from build123d import *

# Parameters (mm, degrees)
SKETCH1_W           = 13
SKETCH1_H           = 13
BOSS_EXTRUDE1_DEPTH = 85
SKETCH2_W           = 13
SKETCH2_H           = 30.5
BOSS_EXTRUDE2_DEPTH = 3
SKETCH3_R           = 2.1
CUT_EXTRUDE1_DEPTH  = 11.5
SKETCH4_R           = 5.25
CUT_EXTRUDE2_DEPTH  = 4.5


with BuildPart() as part:
    # Sketch1 → Boss-Extrude1 (new, symmetric)
    with BuildSketch(Plane.XY):
        Rectangle(SKETCH1_W, SKETCH1_H)
    extrude(amount=BOSS_EXTRUDE1_DEPTH, both=True)

    # Sketch2 → Boss-Extrude2 (add, symmetric)
    with BuildSketch(Plane.XY.offset(82)):
        with Locations((0, -20.75)):
            Rectangle(SKETCH2_W, SKETCH2_H)
    extrude(amount=BOSS_EXTRUDE2_DEPTH, both=True)

    # Sketch3 → Cut-Extrude1 (cut, symmetric)
    with BuildSketch(Plane(origin=(0, 0, 0), x_dir=(0, 0, -1), z_dir=(1, 0, 0))):
        with Locations((72.5, 0)):
            Circle(SKETCH3_R)
        with Locations((47.5, 0)):
            Circle(SKETCH3_R)
        with Locations((22.5, 0)):
            Circle(SKETCH3_R)
        with Locations((-2.5, 0)):
            Circle(SKETCH3_R)
        with Locations((-27.5, 0)):
            Circle(SKETCH3_R)
        with Locations((-52.5, 0)):
            Circle(SKETCH3_R)
        with Locations((-72.5, 0)):
            Circle(SKETCH3_R)
    extrude(amount=CUT_EXTRUDE1_DEPTH, both=True, mode=Mode.SUBTRACT)

    # Sketch4 → Cut-Extrude2 (cut, symmetric)
    with BuildSketch(Plane(origin=(-6.5, 0, 0), x_dir=(0, 0, -1), z_dir=(1, 0, 0))):
        with Locations((72.5, 0)):
            Circle(SKETCH4_R)
        with Locations((47.5, 0)):
            Circle(SKETCH4_R)
        with Locations((22.5, 0)):
            Circle(SKETCH4_R)
        with Locations((-2.5, 0)):
            Circle(SKETCH4_R)
        with Locations((-27.5, 0)):
            Circle(SKETCH4_R)
        with Locations((-52.5, 0)):
            Circle(SKETCH4_R)
        with Locations((-72.5, 0)):
            Circle(SKETCH4_R)
    extrude(amount=CUT_EXTRUDE2_DEPTH, both=True, mode=Mode.SUBTRACT)


solid = part.part
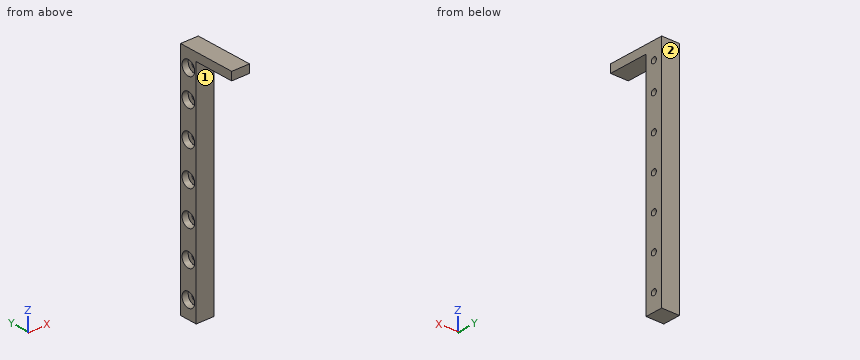
The listing builds one solid part. Answer for the finished solid, in the listing's coordinates (mm). Face numbers are marked on the shaded views. A direction names the side the tool comes from. Give positions to 0.01 mm unless a question says otherwise; leave off trailing zeros. Write each loop counter-clockwise with the first axis right and the second up, starting at its lowest first coordinate (ties: lowest second). Pieces come first, ordered by that corner, then holes. Notation, with made-up numbers: (36.25, 40) - (92.25, 40) arc R17 cw to (92.25, 65) - close; hole circle Ø8 at (-26.75, 81.25). An arc over 180 degrees is marked (long way). One line per question, with ' | ' between items. Start each with the question number.
1. Given P1, Ø4, axis at x = 1.5, z = 8.5, coming from the -Y side; P2, Ø5.5, axis at y = 0, z = 2.5, coming from the -X side, each flat-ended and moving along its own axis, determine where each tip first touches the part or whether it passes through.
2. Section C-C, the plane y = 0 is taken. Count the separate pieces of the cut face and the enclosed holes in it, then the cut area to 3 significant figures.
3. Straight lines are drawn through the part: line 1 (Y direction, x = 1, z = -72.5); line 2 (Y direction, x = 4, z = -65.5); line 3 (Y direction, x = -4.8, z = 52.5). For each, find the intervals that lie inside material, in ascending order.
4. Section D-D, the plane y = -14 is taken. Determine the outline of the cut face in (x, z).
5. For the marked faces 1 and 2, determine the directions among +Z, -Z, +X, -X, +Y, -Y from which every point of the face is accessible in a straight line to the end or side of a thin tool.
6. Section B-B, the plane x = 3.5 is taken. Determine the outline of the cut face in (y, z).
7. Section A-A, the plane z = 27.5 is taken. Determine the outline of the cut face in (x, y).
Result:
1) P1: stops at y = -6.5 | P2: stops at x = -2
2) separate pieces: 8 | enclosed holes: 0 | area: 1,630 mm2
3) line 1: y = -6.5 to -2.1, 2.1 to 6.5 | line 2: y = -6.5 to 6.5 | line 3: y = -6.5 to -5.25, 5.25 to 6.5
4) outline: (-6.5, 79) - (6.5, 79) - (6.5, 85) - (-6.5, 85) - close
5) face 1: -Z, +X, -X, -Y | face 2: +Z, -Z, +X, -X, +Y
6) outline: (-36, 79) - (-6.5, 79) - (-6.5, -85) - (6.5, -85) - (6.5, 85) - (-36, 85) - close; hole circle Ø4.2 at (0, -72.5); hole circle Ø4.2 at (0, -47.5); hole circle Ø4.2 at (0, -22.5); hole circle Ø4.2 at (0, 2.5); hole circle Ø4.2 at (0, 27.5); hole circle Ø4.2 at (0, 52.5); hole circle Ø4.2 at (0, 72.5)
7) outline: (-6.5, -6.5) - (6.5, -6.5) - (6.5, -2.1) - (-2, -2.1) - (-2, -5.25) - (-6.5, -5.25) - close; (-6.5, 5.25) - (-2, 5.25) - (-2, 2.1) - (6.5, 2.1) - (6.5, 6.5) - (-6.5, 6.5) - close
